Could you check a few things on this drawing? It's one solid part, dimensions in mm from its lowest x, y, z. A direction names the side the tool comes from. Give positions to 0.01 mm unless a question says otherwise; leave off trailing zeros. Order: outer loops, then holes, each group sorted by start corner. A loop starts at its lowest first (then second) coordinate and runs counter-clockwise, first axis right, second up. Notation, with made-up numbers: M 58,0 L 113,0 A34 ccw 113,33 Z; hole C -35.75,31 d4. An arc over 180 degrees is marked long. Use one line per item in the form item = value. Start each with the question number.
1. For the marked faces 1 and 2, which set-ups out of +Z, -Z, +X, -X, +Y, -Y let a thin tool reach every point of the face, with its end or its side?
2. I want a section at A-A, the plane x = 12.5. List the corners of the cut face in (y, z) for me.
3. We'd pull the mould along Z, two halves only. Please class the marked faces 3, 4 and 5: +Z half, -Z half, draft (parallel to the pull), parting line (faces both ways), or undercut.
4. I want a section at D-D, the plane z = 41.5. List the corners of the cut face in (x, y) for me.
5. I need wall thicknesses on L1, parallel to Z at x = 3.5, y = 58; L2, parallel to Z at x = 12, y = 57; L3, parallel to Z at x = 7.75, y = 57.5 (1 decimal). Which ranges of each line are inside material? Lowest first, please.
6. Will these pins go through, and if not, where does the flat tip stop? P1, Ø4.5, axis at y = 56.79, z = 65, coming from the +X side; P2, Ø5, axis at x = 13, z = 26.5, coming from the -Y side; P3, Ø1, axis at x = 7, y = 64, coming from the +Z side (1 decimal); P4, Ø8, axis at x = 4, z = 48.5, coming from the +Y side (1 decimal).
7. I want a section at C-C, the plane z = 5. List the corners of the cut face in (x, y) for me.
8. I want a section at B-B, the plane y = 17.5. List the corners of the cut face in (x, z) for me.
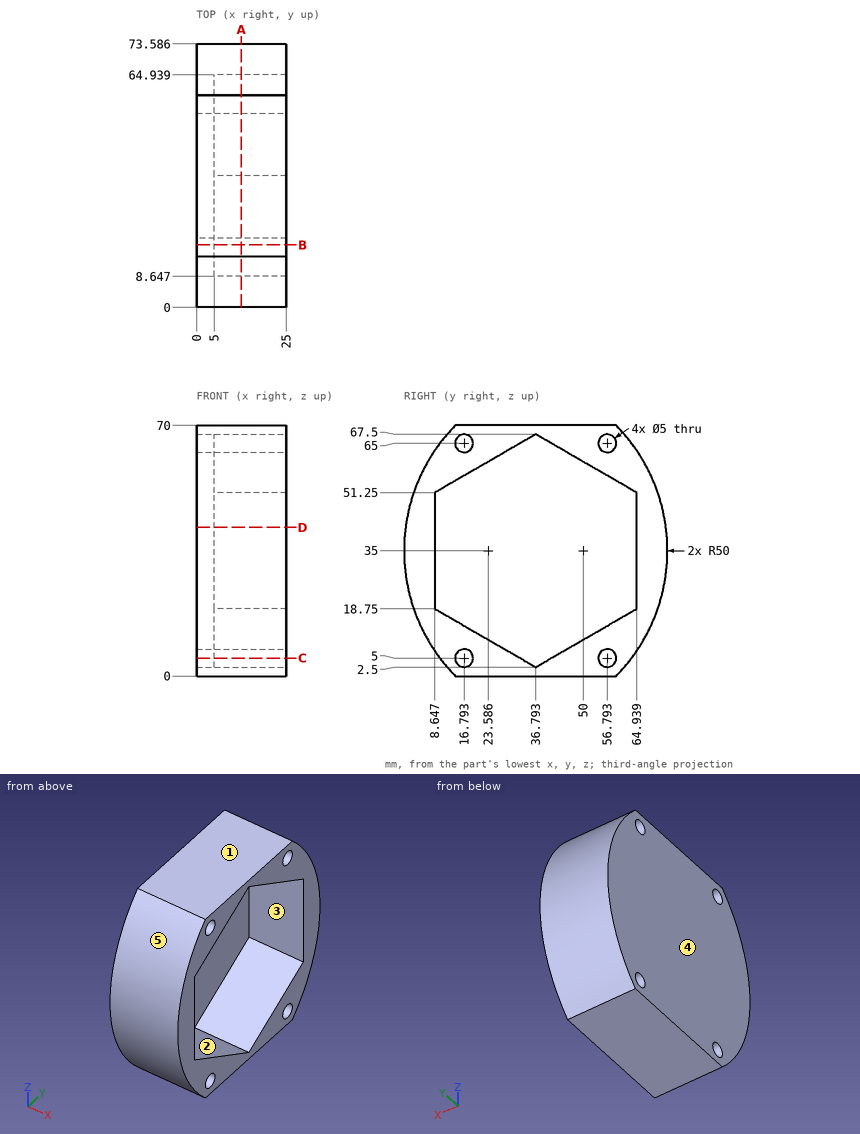
Check result:
q1.face_1 = +Z, +X, -X, +Y, -Y
q1.face_2 = +X
q2.outline = M 14.29,0 L 59.29,0 A50 ccw 59.29,70 L 14.29,70 A50 ccw Z; hole M 8.65,18.75 L 36.79,2.5 L 64.94,18.75 L 64.94,51.25 L 36.79,67.5 L 8.65,51.25 Z; hole C 16.79,5 d5; hole C 16.79,65 d5; hole C 56.79,5 d5; hole C 56.79,65 d5
q3.face_3 = undercut
q3.face_4 = draft
q3.face_5 = parting line
q4.outline = M 0,0.42 L 25,0.42 L 25,8.65 L 5,8.65 L 5,64.94 L 25,64.94 L 25,73.16 L 0,73.16 Z
q5.L1 = 0 to 2.81, 7.19 to 62.81, 67.19 to 70
q5.L2 = 0 to 2.51, 7.49 to 14.17, 55.83 to 62.51, 67.49 to 70
q5.L3 = 0 to 2.6, 7.4 to 14.5, 55.5 to 62.6, 67.4 to 70
q6.P1 = through
q6.P2 = 0.36
q6.P3 = 65.1
q6.P4 = 72.7
q7.outline = M 0,10 L 25,10 L 25,14.29 L 0,14.29 Z; M 0,19.29 L 25,19.29 L 25,32.46 L 5,32.46 L 5,41.12 L 25,41.12 L 25,54.29 L 0,54.29 Z; M 0,59.29 L 25,59.29 L 25,63.59 L 0,63.59 Z
q8.outline = M 0,0 L 25,0 L 25,2.6 L 0,2.6 Z; M 0,7.4 L 25,7.4 L 25,13.64 L 5,13.64 L 5,56.36 L 25,56.36 L 25,62.6 L 0,62.6 Z; M 0,67.4 L 25,67.4 L 25,70 L 0,70 Z
